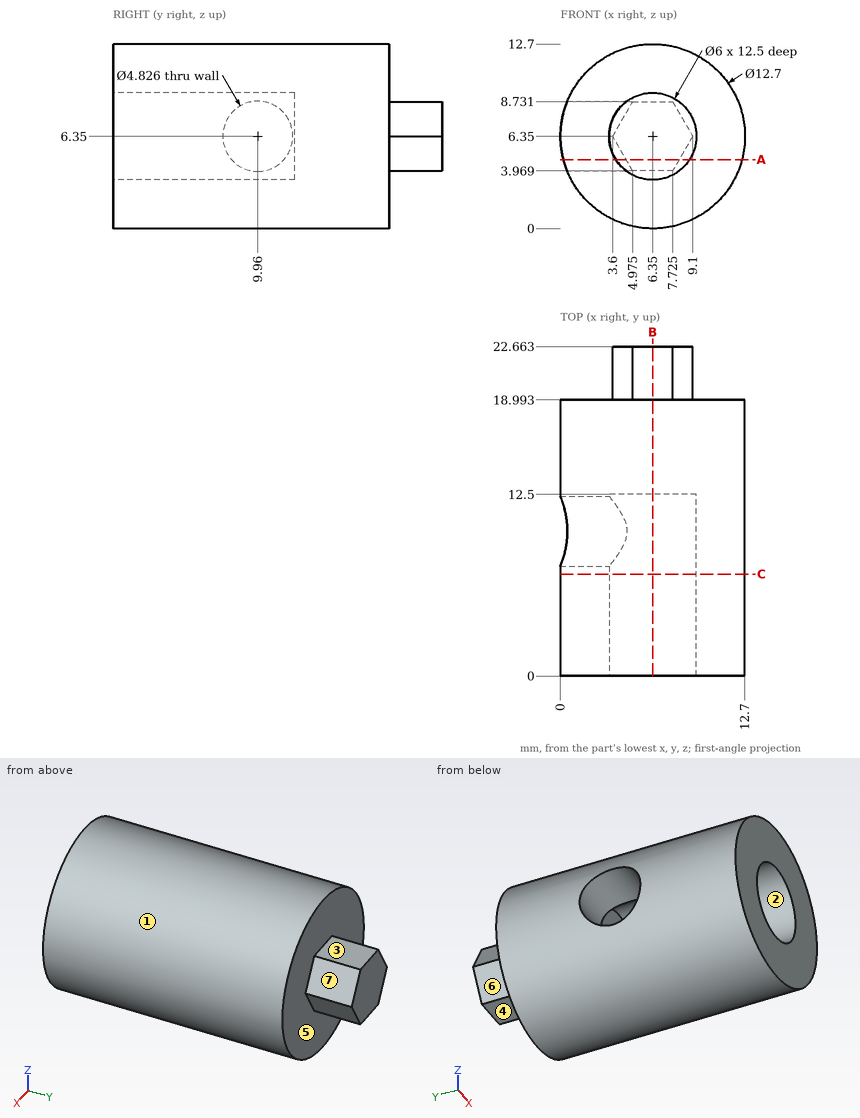
Can you work these out from the drawing? Everything is in mm from the part's minimum corner. A direction names the side the tool comes from. Coordinates: 2 decimals unless noted, no trailing zeros. Write each loop counter-clockwise with the first axis right and the second up, starting at its lowest first coordinate (ties: lowest second). Pieces come first, ordered by that corner, then holes. Notation, with made-up numbers: (60, -27) -> (70, -27) arc R30 cw to (70, 7) -> close; hole circle Ø10 at (58.25, -17.75). An arc over 180 degrees is marked (long way). Write item = value, one per line.
(1) On a 3-axis mill with a long thin cutter (end or side, diameter ignored), from which of +Z, -Z, +X, -X, +Y, -Y can I reach the whole of each face in a straight line? I mean the marked faces 4, 5, 6 and 7. Say none if no direction works.
Verdict:
face_4 = -Z, +X, -X, +Y
face_5 = +Y
face_6 = -Z, -X, +Y
face_7 = +Z, +X, +Y
(2) Imagine slicing it at B-B (x = 6.35). Please give me the cut outline in (y, z).
Verdict:
outline = (0, 0) -> (18.99, 0) -> (18.99, 3.97) -> (22.66, 3.97) -> (22.66, 8.73) -> (18.99, 8.73) -> (18.99, 12.7) -> (0, 12.7) -> (0, 9.35) -> (12.5, 9.35) -> (12.5, 3.35) -> (0, 3.35) -> close
(3) Imagine slicing it at A-A (z = 4.75). Please give me the cut outline in (x, y) (1 decimal), and give its area (3 significant figures).
Verdict:
outline = (0.2, 0) -> (3.8, 0) -> (3.8, 8.2) -> (0.2, 8.2) -> close; (0.2, 11.8) -> (3.8, 11.8) -> (3.8, 12.5) -> (8.9, 12.5) -> (8.9, 0) -> (12.5, 0) -> (12.5, 19) -> (8.2, 19) -> (8.2, 22.7) -> (4.5, 22.7) -> (4.5, 19) -> (0.2, 19) -> close
area = 170 mm^2
(4) If I drill on probe 1 along Y at (x, z) = (7.75, 12); probe 2 along Z at (x, y) = (1, 8) (1 decimal); probe 3 along Y at (x, z) = (7.75, 8.25), over which ranges is the centre line in solid material (lowest first)?
Verdict:
probe_1 = 0 to 18.99
probe_2 = 2.9 to 4.9, 7.8 to 9.8
probe_3 = 12.5 to 22.66
(5) Thinking about a two-plate mould opening in Z: for the marked faces 1, 2 and 3, which applies, +Z half, -Z half, draft (parallel to the pull), parting line (faces both ways), or undercut?
Verdict:
face_1 = parting line
face_2 = undercut
face_3 = +Z half
(6) Imagine slicing it at C-C (y = 7). Please give me the cut outline in (x, z).
Verdict:
outline = circle Ø12.7 at (6.35, 6.35); hole circle Ø6 at (6.35, 6.35)
(7) For pin 1 (0.8 mm diameter, centred on x = 7, y = 20.5, fed in from +Z); pin 2 (4.5 mm diameter, centred on y = 9.96, z = 6.35, fed in from -X) (1 decimal); pin 3 (1.5 mm diameter, centred on x = 11, z = 2, fed in from +Y), each with a flat end and sliding along its axis, tell me the tip position at first contact or that it passes through.
Verdict:
pin_1 = 8.73
pin_2 = 8.3
pin_3 = 18.99
